```python
from build123d import *

# Parameters (mm, degrees)
SKETCH004_W     = 28
SKETCH004_H     = 31
PAD001_DEPTH    = 2
SKETCH005_R     = 2.75
PAD002_DEPTH    = 2.4
SKETCH006_R     = 1.6
HOLE001_DEPTH   = 25
SKETCH_W        = 10
SKETCH_H        = 9
POCKET_DEPTH    = 5
FILLET_R        = 2
SKETCH007_W     = 8.5
SKETCH007_H     = 3.5
POCKET001_DEPTH = 2
FILLET001_R     = 0.5


with BuildPart() as part:
    # Sketch004 → Pad001 (new body)
    with BuildSketch(Plane.XY):
        with Locations((-14, -15.5)):
            Rectangle(SKETCH004_W, SKETCH004_H)
    extrude(amount=PAD001_DEPTH)

    # Sketch005 (on Face6 of Pad001) → Pad002 (join)
    with BuildSketch(Plane.XY.offset(2)):
        with Locations((-22.5, -5.5)):
            Circle(SKETCH005_R)
        with Locations((-5.5, -5.5)):
            Circle(SKETCH005_R)
        with Locations((-22.5, -25.5)):
            Circle(SKETCH005_R)
        with Locations((-5.5, -25.5)):
            Circle(SKETCH005_R)
    extrude(amount=PAD002_DEPTH)

    # Sketch006 (on Face4 of Pad002) → Hole001 (cut)
    with BuildSketch(Plane(origin=(0, 0, 0), x_dir=(1, 0, 0), z_dir=(0, 0, -1))):
        with Locations((-22.5, 25.5)):
            Circle(SKETCH006_R)
        with Locations((-5.5, 25.5)):
            Circle(SKETCH006_R)
        with Locations((-5.5, 5.5)):
            Circle(SKETCH006_R)
        with Locations((-22.5, 5.5)):
            Circle(SKETCH006_R)
    extrude(amount=-HOLE001_DEPTH, mode=Mode.SUBTRACT)

    # Sketch (on Face5 of Hole001) → Pocket (cut)
    with BuildSketch(Plane.XY.offset(2)):
        with Locations((-14, -26.5)):
            Rectangle(SKETCH_W, SKETCH_H)
    extrude(amount=-POCKET_DEPTH, mode=Mode.SUBTRACT)

    # Fillet
    fillet_edges = [part.edges().sort_by_distance(p)[0] for p in [
        (0, 0, 1),
        (0, -31, 1),
        (-28, 0, 1),
        (-28, -31, 1),
    ]]
    fillet(fillet_edges, radius=FILLET_R)

    # Sketch007 (on Face5 of Fillet) → Pocket001 (cut)
    with BuildSketch(Plane.XY.offset(2)):
        with Locations((-14, -8.5)):
            Rectangle(SKETCH007_W, SKETCH007_H)
    extrude(amount=-POCKET001_DEPTH, mode=Mode.SUBTRACT)

    # Fillet001
    fillet001_edges = [part.edges().sort_by_distance(p)[0] for p in [
        (-9.75, -6.75, 1),
        (-9.75, -10.25, 1),
        (-18.25, -10.25, 1),
        (-18.25, -6.75, 1),
    ]]
    fillet(fillet001_edges, radius=FILLET001_R)


solid = part.part
```
For this review, take the finished solid that the model builds, in its own axes (mm). A direction names the side the tool comes from. Round coordinates to 2 decimals unless told otherwise and drop trailing zeros. Loops run counter-clockwise (first coordinate to the right, second up) from the corner with the lowest first, then second, coordinate; pieces in that order, holes last.
Q1. Add section C-C on y = -5.5. Write out the cut boundary in (x, z), plus the area to 3 significant figures.
Result sheet:
outline: (-28, 0) - (-24.1, 0) - (-24.1, 4.4) - (-25.25, 4.4) - (-25.25, 2) - (-28, 2) - close; (-20.9, 0) - (-7.1, 0) - (-7.1, 4.4) - (-8.25, 4.4) - (-8.25, 2) - (-19.75, 2) - (-19.75, 4.4) - (-20.9, 4.4) - close; (-3.9, 0) - (0, 0) - (0, 2) - (-2.75, 2) - (-2.75, 4.4) - (-3.9, 4.4) - close
area: 54.2 mm2
Q2. Add section D-D on x = -17. Write out the cut boundary in (y, z), plus the area to 3 significant figures.
Result sheet:
outline: (-22, 0) - (-10.25, 0) - (-10.25, 2) - (-22, 2) - close; (-6.75, 0) - (0, 0) - (0, 2) - (-6.75, 2) - close
area: 37.0 mm2
Q3. Insertion check: pin 1 Ø1 at (x, y) = (-24.5, -19) entering from +Z; pin 2 Ø2 at (x, z) = (-14, 1.5) entering from -Y. Each pin has a flat end and moves straight along its axis. Give the tip position at first contact, or say it passes through.
Result sheet:
pin 1: stops at z = 2
pin 2: stops at y = -22
Q4. Add section A-A on z = 3.9. Write out the cut boundary in (x, y).
Result sheet:
outline: circle Ø5.5 at (-22.5, -25.5); circle Ø5.5 at (-22.5, -5.5); circle Ø5.5 at (-5.5, -25.5); circle Ø5.5 at (-5.5, -5.5); hole circle Ø3.2 at (-22.5, -25.5); hole circle Ø3.2 at (-22.5, -5.5); hole circle Ø3.2 at (-5.5, -25.5); hole circle Ø3.2 at (-5.5, -5.5)
Q5. Mouldability with a two-part tool opening along X and no side actions: class faces 5 (the face through (-0.6, -0.57, 1.01)), 6 (the face through (-14, -6.75, 1)), 7 (the face through (-23, -31, 1)) as +X half, -X half, draft (parallel to the pull), parting line (faces both ways), or undercut.
Result sheet:
face 5: +X half
face 6: undercut
face 7: draft
Q6. Machinability: for faces 1 (the face through (-14, -10.25, 1)), 2 (the face through (-9, -27, 1)), 3 (the face through (-5.858, -22.773, 3.183)), 4 (the face through (-4, -7, 4.4)), which of the approach directions +Z, -Z, +X, -X, +Y, -Y give a long, thin tool a straight path to every point of the face, cutting with its end or side? Answer none if there is none.
Result sheet:
face 1: +Z, -Z
face 2: +Z, -Z, -Y
face 3: +Z
face 4: +Z, +X, -X, +Y, -Y
Q7. To check wall thickness, follow line 1 along Y through (x, z) = (-22.5, 1.1); line 2 along X through (y, z) = (-25.5, 1.4); line 3 along X through (y, z) = (-5.5, 1.7). State the ranges of each line that lie inside material, in increasing order.
Result sheet:
line 1: y = -31 to -27.1, -23.9 to -7.1, -3.9 to 0
line 2: x = -28 to -24.1, -20.9 to -19, -9 to -7.1, -3.9 to 0
line 3: x = -28 to -24.1, -20.9 to -7.1, -3.9 to 0
Q8. Add section B-B on x = -22.5. Write out the cut boundary in (y, z), plus the area to 3 significant figures.
Result sheet:
outline: (-31, 0) - (-27.1, 0) - (-27.1, 4.4) - (-28.25, 4.4) - (-28.25, 2) - (-31, 2) - close; (-23.9, 0) - (-7.1, 0) - (-7.1, 4.4) - (-8.25, 4.4) - (-8.25, 2) - (-22.75, 2) - (-22.75, 4.4) - (-23.9, 4.4) - close; (-3.9, 0) - (0, 0) - (0, 2) - (-2.75, 2) - (-2.75, 4.4) - (-3.9, 4.4) - close
area: 60.2 mm2
